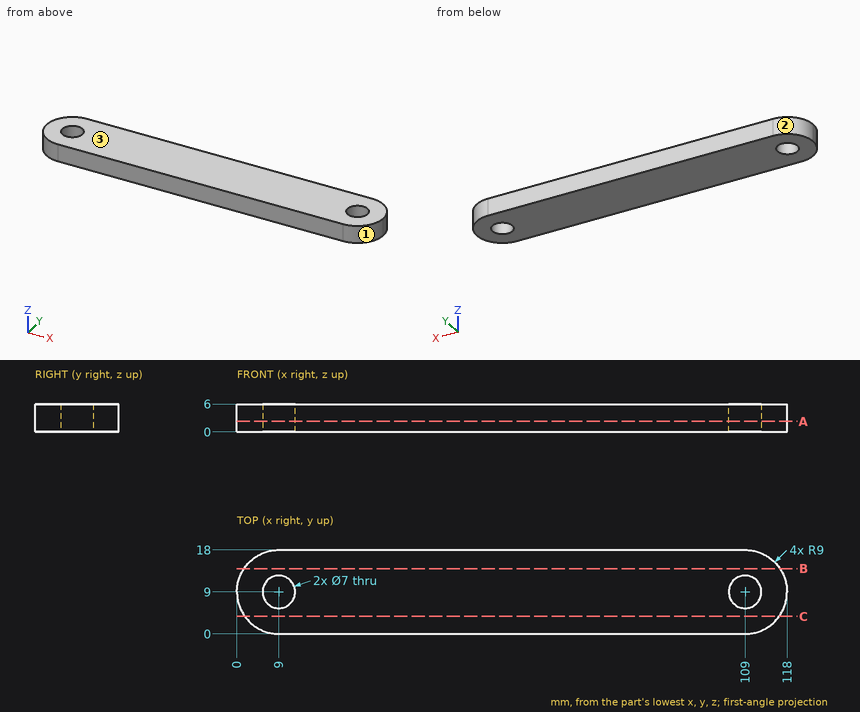
Could you check a few things on this drawing? It's one solid part, dimensions in mm from its lowest x, y, z. Give positions to 0.01 mm unless a question says otherwise; leave off trailing zeros. Order: outer loops, then holes, each group sorted by start corner. A loop starts at its lowest first (then second) coordinate and runs counter-clockwise, first axis right, second up. Notation, with made-up numbers: M 36,62.25 L 51,62.25 A23 cw 51,99.25 Z; hole C 47.25,9 d4. An arc over 180 degrees is marked long. Use one line per item in the form item = value. Start each with the question number.
Item 1: If we section it at A-A (z = 2.25): State how many separate pieces and enclosed holes the cut face has, then the cut area to 3 significant figures.
Item 2: If we section it at B-B (y = 14): Write out the boundary of the cut face in (x, z).
Item 3: If we section it at C-C (y = 3.75): Write out the boundary of the cut face in (x, z).
Item 4: If I drill on line 1 along X through (y, z) = (8.75, 3.8); line 2 along Y through (x, z) = (9, 4.5); line 3 along X through (y, z) = (6.5, 0.55), over which ranges is the centre line in solid material (lowest first)?
Item 5: We'd pull the mould along X, two halves only. Please class the marked faces 1, 2 and 3: +X half, -X half, draft (parallel to the pull), parting line (faces both ways), or undercut.
Outcome:
q1.separate_pieces = 1
q1.enclosed_holes = 2
q1.area = 1,980 mm2
q2.outline = M 1.52,0 L 116.48,0 L 116.48,6 L 1.52,6 Z
q3.outline = M 1.69,0 L 116.31,0 L 116.31,6 L 1.69,6 Z
q4.line_1 = 0 to 5.51, 12.49 to 105.51, 112.49 to 118
q4.line_2 = 0 to 5.5, 12.5 to 18
q4.line_3 = 0.35 to 6.55, 11.45 to 106.55, 111.45 to 117.65
q5.face_1 = +X half
q5.face_2 = -X half
q5.face_3 = draft
